CAD build for the part. Positions are in the model's coordinates, mm. A direction names the side the tool comes from. Coordinates: 2 decimals unless noted, no trailing zeros. Loops run counter-clockwise (first coordinate to the right, second up) from the corner with the lowest first, then second, coordinate; pieces in that order, holes last. Notation, with made-up numbers: (21.25, 63.25) -> (46.25, 63.25) arc R25 ccw to (46.25, 83.25) -> close; hole circle Ø2 at (-14.5, 44). An arc over 180 degrees is marked (long way). Return JSON: item names as keys, results as strings. Group by question number.
(1) Saw through at D-D on y = 0.3. Write the cut outline in (x, z) (1 decimal), then the cut area to 3 significant figures.
(2) Saw through at A-A on x = 0. Write the cut outline in (y, z), then the cut area to 3 significant figures.
(3) Saw through at C-C on x = 17. Write the cut outline in (y, z).
(4) Tool access for faces 1 (the face through (0, 1.6, -20)), 2 (the face through (24.764, 0.789, -0.242)): list every direction of +Z, -Z, +X, -X, +Y, -Y with a clear straight run to the whole face (end or side of a thin tool).
(5) Mould opens along Z. For faces 3 (the face through (0, 0, -20)), 4 (the face through (-24.764, 0.789, 0.242)), 5 (the face through (6.607, 0.789, 29.755)) say: pulls with the +Z half, pulls with the -Z half, needs draft (parallel to the pull), parting line crosses it, or undercut.
(6) Flat gauge pin, fed straight in: pin 1 Ø1.9 at (x, z) = (0, 22.25) entering from -Y (3 decimals). Where does the tip first touch, or does it go through?
(7) Saw through at B-B on z = -22.5. Write the cut outline in (x, y), then the cut area to 3 significant figures.
(8) Probe L1, parallel to X at y = 0.5, z = -0.5; L2, parallel to Z at x = 12, y = 0.3; L3, parallel to Z at x = 2, y = 0.5. List the from-to ranges inside material, lowest first.
Autodesk Inventor part; units mm, degrees
ref_plane "YZ Plane" through (0, 0, 0) normal (1, 0, 0) x (0, 1, 0)
ref_plane "XZ Plane" through (0, 0, 0) normal (0, 1, 0) x (-1, 0, 0)
ref_plane "XY Plane" through (0, 0, 0) normal (0, 0, 1) x (1, 0, 0)
sketch "Sketch1" plane through (0, 0, 0) normal (0, 1, 0) x (-1, 0, 0)
  circle A0 centre (0, 0) radius 24.765
  circle A1 centre (0, 0) radius 30.48
  dimension "d0" = 49.53
  dimension "d1" = 60.96
extrude "Extrusion1" add sketch "Sketch1" along normal blind 1.6002
sketch "Sketch2" plane through (0, 1.6002, 0) normal (0, 1, 0) x (1, 0, 0)
  line L0 (0, 0) -> (0, 15.9004)
  line L1 (0, 15.9004) -> (-18.9864, 15.9004)
  circle A0 centre (0, 0) radius 24.765
  line L2 (0, 15.9004) -> (18.9864, 15.9004)
  dimension "d4" = 15.9004
extrude "Extrusion2" add sketch "Sketch2" against normal blind 1.6002 contours L1 A0 L2 picked at (-11.1522, 17.2995)
pattern_circular "Circular Pattern1" count 2 over 360 about axis through (0, 0, 0) along (0, 1, 0) of "Extrusion2"
sketch "Sketch3" plane through (0, 1.6002, 0) normal (0, 1, 0) x (1, 0, 0)
  circle A0 centre (0, 0) radius 30.48
  line L0 (-18.9864, -15.9004) -> (18.9864, -15.9004)
  line L1 (0, 0) -> (0, -22.2504)
  dimension "d11" = 22.2504
hole "Hole1" at (0, 1.6002, 22.2504) direction (0, -1, 0) diameter 3.175 depth 25.4 tip angle 118
pattern_circular "Circular Pattern2" count 2 over 360 about axis through (0, 0, 0) along (0, 1, 0) of "Hole1"
properties part number "retainer"
Geometry results:
{
 "1": {"outline": "circle Ø61 at (0, 0); hole (-19, -15.9) -> (19, -15.9) arc R24.8 ccw to (19, 15.9) -> (-19, 15.9) arc R24.8 ccw to start; hole circle Ø3.2 at (0, -22.3); hole circle Ø3.2 at (0, 22.3)", "area": "1,440 mm²"},
 "2": {"outline": "(0, -30.48) -> (1.6, -30.48) -> (1.6, -23.84) -> (0, -23.84) -> close; (0, -20.66) -> (1.6, -20.66) -> (1.6, -15.9) -> (0, -15.9) -> close; (0, 15.9) -> (1.6, 15.9) -> (1.6, 20.66) -> (0, 20.66) -> close; (0, 23.84) -> (1.6, 23.84) -> (1.6, 30.48) -> (0, 30.48) -> close", "area": "36.5 mm²"},
 "3": {"outline": "(0, -25.3) -> (1.6, -25.3) -> (1.6, -15.9) -> (0, -15.9) -> close; (0, 15.9) -> (1.6, 15.9) -> (1.6, 25.3) -> (0, 25.3) -> close"},
 "4": {"face 1": "+Z, -Z, +X, -X, +Y", "face 2": "+Y, -Y"},
 "5": {"face 3": "needs draft", "face 4": "undercut", "face 5": "parting line crosses it"},
 "6": {"pin 1": "through"},
 "7": {"outline": "(-20.56, 0) -> (-1.57, 0) -> (-1.57, 1.6) -> (-20.56, 1.6) -> close; (1.57, 0) -> (20.56, 0) -> (20.56, 1.6) -> (1.57, 1.6) -> close", "area": "60.8 mm²"},
 "8": {"L1": "-30.48 to -24.76, 24.76 to 30.48", "L2": "-28.02 to -15.9, 15.9 to 28.02", "L3": "-30.41 to -15.9, 15.9 to 30.41"}
}
